Verification items for the finished model (mm, model axes). Coordinates: 2 decimals unless noted, no trailing zeros. Write each loop counter-clockwise with the first axis right and the second up, starting at its lowest first coordinate (ties: lowest second). Pieces come first, ordered by that corner, then holes. Notation, with made-up numbers: M 82.25,44 L 96.25,44 A9 ccw 96.25,55 Z; hole C -27.5,82.5 d1. An arc over 180 degrees is marked long. One line per item, written item: value.
Autodesk Inventor part; units mm, degrees
ref_plane "YZ Plane" through (0, 0, 0) normal (1, 0, 0) x (0, 1, 0)
ref_plane "XZ Plane" through (0, 0, 0) normal (0, 1, 0) x (-1, 0, 0)
ref_plane "XY Plane" through (0, 0, 0) normal (0, 0, 1) x (1, 0, 0)
sketch "Sketch1" plane through (0, 0, 0) normal (0, 0, 1) x (1, 0, 0)
  line L0 (-0.75, 0.15) -> (0.75, 0.15)
  line L1 (0.75, 0.15) -> (0.75, -0.15)
  line L2 (0.75, -0.15) -> (-0.75, -0.15)
  line L3 (-0.75, -0.15) -> (-0.75, 0.15)
  line L4 (0, -0.2204) -> (0, 0)
  line L5 (0, 0) -> (0.3288, 0)
  dimension "d0" = 1.5
  dimension "d1" = 0.3
sketch3d "3D Sketch1"
  line L0 (0, 0, 0) -> (0, 0, 11.4491)
  arc A0 (0, 0, 11.4491) -> (0, 0.4657, 12.2944) centre (0, 1, 11.4491) ccw
  line L1 (0, 0.4657, 12.2944) -> (0, 5.8049, 15.6693)
  arc A1 (0, 5.8049, 15.6693) -> (0, 19, 8.4) centre (0, 10.4, 8.3999) ccw
  line L2 (0, 19, 8.4) -> (0, 19, -8.4)
  arc A2 (0, 19, -8.4) -> (0, 5.8048, -15.6694) centre (0, 10.4, -8.4) ccw
  line L3 (0, 5.8048, -15.6694) -> (0, 0.4657, -12.2944)
  arc A3 (0, 0.4657, -12.2944) -> (0, 0, -11.4491) centre (0, 1, -11.4491) ccw
  line L4 (0, 0, -11.4491) -> (0, 0, 0)
  dimension "d10" = 16.8
  dimension "d11" = 12
  dimension "d12" = 12
  dimension "d13" = 19
  dimension "d2" = 8.6
  dimension "d3" = 8.6
  dimension "d5" = 1
  dimension "d6" = 1
sweep "Sweep1" add profiles "Sketch1" path "3D Sketch1"
sketch "Sketch2" plane through (0, 0, 0) normal (1, 0, 0) x (0, 1, 0)
  line L0 (17.8246, 14.4103) -> (17.1175, 13.7032)
  line L1 (17.1175, 13.7032) -> (15.7033, 15.1174)
  line L2 (15.7033, 15.1174) -> (16.4104, 15.8245)
  line L3 (16.4104, 15.8245) -> (17.8246, 14.4103)
  arc A0 (18.85, 8.4) -> (5.8851, 15.5425) centre (10.4, 8.3999) ccw
  line L4 (10.4, 8.3999) -> (24.1814, 22.1813) construction
  line L5 (-0.15, -11.4491) -> (-0.15, 11.4491) construction
  point P0 (0, 0)
  point P1 (16.4104, 14.4103)
  point P2 (16.4104, 14.4103)
  dimension "d15" = 2
  dimension "d16" = 1
  dimension "d17" = 45
  dimension "d18" = 8.5
extrude "Extrusion1" add sketch "Sketch2" along normal mid plane 2
equation "\"d6\" = d5"
properties part number "battery_cord_2x" material "Polyester Yarn"
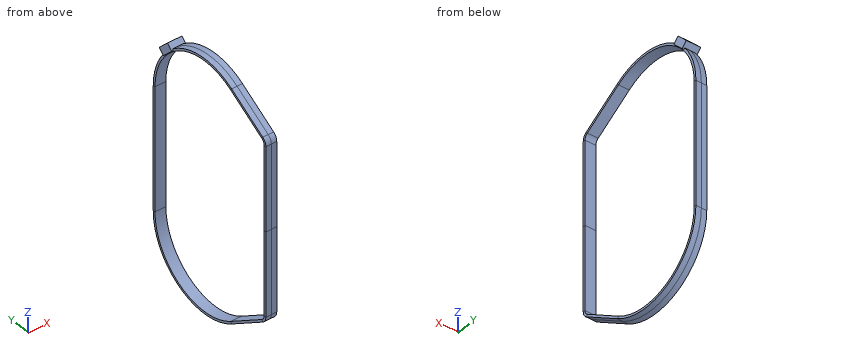
Item 1: Cross-section at B-B, the plane y = 11.25. Enter the section's corners in (x, z).
The answers:
outline: M -0.75,-17.11 L 0.75,-17.11 L 0.75,-16.81 L -0.75,-16.81 Z; M -0.75,16.81 L 0.75,16.81 L 0.75,17.11 L -0.75,17.11 Z
Item 2: Cross-section at A-A, the plane z = 4.5. Enter the section's corners in (x, y), and give its area (3 significant figures).
The answers:
outline: M -0.75,-0.15 L 0.75,-0.15 L 0.75,0.15 L -0.75,0.15 Z; M -0.75,18.85 L 0.75,18.85 L 0.75,19.15 L -0.75,19.15 Z
area: 0.900 mm²
Item 3: Cross-section at C-C, the plane x = -0.3. Enter the section's corners in (y, z), and give its area (3 significant figures).
The answers:
outline: M -0.15,-11.45 A1.15 ccw 0.39,-12.42 L 5.72,-15.8 A8.75 ccw 19.15,-8.4 L 19.15,8.4 A8.75 ccw 17.25,13.84 L 17.82,14.41 L 16.41,15.82 L 15.84,15.25 A8.75 ccw 5.72,15.8 L 0.39,12.42 A1.15 ccw -0.15,11.45 Z; hole M 0.15,-11.45 A0.85 ccw 0.55,-12.17 L 5.88,-15.54 A8.45 ccw 18.85,-8.4 L 18.85,8.4 A8.45 ccw 5.89,15.54 L 0.55,12.17 A0.85 ccw 0.15,11.45 Z
area: 28.9 mm²
Item 4: Scan lines: line 1 (Y direction, x = -0.45, z = 4.5); line 2 (Z direction, x = 0.4, y = 4.75); line 3 (Z direction, x = -0.55, y = 10). Record each from-to range of solid material in increasing order.
The answers:
line 1: y = -0.15 to 0.15, 18.85 to 19.15
line 2: z = -15.18 to -14.83, 14.83 to 15.18
line 3: z = -17.14 to -16.84, 16.84 to 17.14
Item 5: Go/stop test with flat-tipped pins: P1, Ø1.1, axis at y = 3.5, z = -14, coming from the +X side; P2, Ø7, axis at y = 14.5, z = -12, coming from the -X side; P3, Ø7, axis at y = 15.5, z = 13, coming from the -X side; P4, Ø3, axis at y = 3, z = -5, coming from the -X side. Record where each tip stops, or that it passes through.
The answers:
P1: stops at x = 0.75
P2: stops at x = -0.75
P3: stops at x = -1
P4: passes through
